```python
from build123d import *

# Parameters (mm, degrees)
SKETCH1_W           = 24.83
SKETCH1_H           = 23.79
BOSS_EXTRUDE1_DEPTH = 1.05
BOSS_EXTRUDE2_DEPTH = 4.5
SKETCH3_W           = 21.41
SKETCH3_H           = 4.84
BOSS_EXTRUDE3_DEPTH = 2.68
SKETCH4_R           = 6.265
BOSS_EXTRUDE4_DEPTH = 2.7
SKETCH5_R           = 5
BOSS_EXTRUDE5_DEPTH = 2
SKETCH6_R           = 7.16
BOSS_EXTRUDE6_DEPTH = 3
SKETCH7_R           = 6
BOSS_EXTRUDE7_DEPTH = 0.1
DOME2_FACE_RADIUS   = 6
DOME2_HEIGHT        = 1


with BuildPart() as part:
    # Sketch1 → Boss-Extrude1 (new body)
    with BuildSketch(Plane(origin=(0, 0, 0), x_dir=(1, 0, 0), z_dir=(0, 1, 0))):
        with Locations((12.415, 11.895)):
            Rectangle(SKETCH1_W, SKETCH1_H)
    extrude(amount=BOSS_EXTRUDE1_DEPTH)

    # Sketch2 → Boss-Extrude2 (add)
    with BuildSketch(Plane(origin=(0, 1.05, 0), x_dir=(1, 0, 0), z_dir=(0, 1, 0))):
        with BuildLine():
            Line((3.745, 17.925), (5.65, 17.925))
            Line((5.65, 17.925), (5.65, 22.44))
            Line((5.65, 22.44), (19.18, 22.44))
            Line((19.18, 22.44), (19.18, 17.92))
            Line((19.18, 17.92), (21.085, 17.92))
            ThreePointArc((21.085, 17.92), (23.335, 15.67), (21.085, 13.42))
            Line((21.085, 13.42), (19.18, 13.42))
            Line((19.18, 13.42), (19.18, 8.91))
            Line((19.18, 8.91), (5.65, 8.91))
            Line((5.65, 8.91), (5.65, 13.425))
            Line((5.65, 13.425), (3.745, 13.425))
            ThreePointArc((3.745, 13.425), (1.495, 15.675), (3.745, 17.925))
        make_face()
    extrude(amount=BOSS_EXTRUDE2_DEPTH)

    # Sketch3 → Boss-Extrude3 (add)
    with BuildSketch(Plane(origin=(0, 1.05, 0), x_dir=(1, 0, 0), z_dir=(0, 1, 0))):
        with Locations((12.415, 2.92)):
            Rectangle(SKETCH3_W, SKETCH3_H)
    extrude(amount=BOSS_EXTRUDE3_DEPTH)

    # Sketch4 → Boss-Extrude4 (add)
    with BuildSketch(Plane(origin=(0, 5.55, 0), x_dir=(1, 0, 0), z_dir=(0, 1, 0))):
        with Locations(Location((12.415, 15.675, 0), (0, 0, 90))):
            Circle(SKETCH4_R)
    extrude(amount=BOSS_EXTRUDE4_DEPTH)

    # Sketch5 → Boss-Extrude5 (add)
    with BuildSketch(Plane(origin=(0, 8.25, 0), x_dir=(1, 0, 0), z_dir=(0, 1, 0))):
        with Locations(Location((12.415, 15.675, 0), (0, 0, 270))):
            Circle(SKETCH5_R)
    extrude(amount=BOSS_EXTRUDE5_DEPTH)

    # Sketch6 → Boss-Extrude6 (add)
    with BuildSketch(Plane(origin=(0, 10.25, 0), x_dir=(1, 0, 0), z_dir=(0, 1, 0))):
        with Locations(Location((12.415, 15.675, 0), (0, 0, 270))):
            Circle(SKETCH6_R)
    extrude(amount=BOSS_EXTRUDE6_DEPTH)

    # Sketch7 → Boss-Extrude7 (add)
    with BuildSketch(Plane(origin=(0, 13.25, 0), x_dir=(1, 0, 0), z_dir=(0, 1, 0))):
        with Locations(Location((12.415, 15.675, 0), (0, 0, 270))):
            Circle(SKETCH7_R)
    extrude(amount=BOSS_EXTRUDE7_DEPTH)

    # Dome2: a dome of height H over a round flat face of radius A is a cap of a sphere of radius (A * A + H * H) / (2 * H)
    dome2_r = (DOME2_FACE_RADIUS * DOME2_FACE_RADIUS + DOME2_HEIGHT * DOME2_HEIGHT) / (2 * DOME2_HEIGHT)
    dome2_base = Plane((12.415, 13.35, -15.675), z_dir=(0, 1, 0))
    with Locations(dome2_base.offset(DOME2_HEIGHT - dome2_r)):
        dome2_ball = Sphere(dome2_r, mode=Mode.PRIVATE)
    add(split(dome2_ball, bisect_by=dome2_base, keep=Keep.TOP, mode=Mode.PRIVATE))


solid = part.part
```
Check sheet for the modelled part. Datum: model origin and axes. Units: mm. A direction names the side the tool comes from. Coordinates: 2 decimals unless noted, no trailing zeros. Loops run counter-clockwise (first coordinate to the right, second up) from the corner with the lowest first, then second, coordinate; pieces in that order, holes last. Notation, with made-up numbers: M -4.5,10.5 L 42.5,10.5 A14 ccw 42.5,21.5 Z; hole C 48.25,-17.5 d5. An arc over 180 degrees is marked long. Answer as a JSON object with one key per item and string values.
1. Sectioned sample at D-D on z = -20. Record the cut outline in (x, y) (3 decimals), and give its area (3 significant figures).
Outcome:
{"outline": "M 0,0 L 24.83,0 L 24.83,1.05 L 19.18,1.05 L 19.18,5.55 L 16.948,5.55 L 16.948,8.25 L 14.924,8.25 L 14.924,10.25 L 18.121,10.25 L 18.121,13.25 L 16.574,13.25 L 16.574,13.35 A17.987 ccw 8.256,13.35 L 8.256,13.25 L 6.709,13.25 L 6.709,10.25 L 9.906,10.25 L 9.906,8.25 L 7.882,8.25 L 7.882,5.55 L 5.65,5.55 L 5.65,1.05 L 0,1.05 Z", "area": "159 mm²"}
2. Sectioned sample at C-C on x = 9.5. Record the cut outline in (y, z) (3 decimals).
Outcome:
{"outline": "M 0,-23.79 L 1.05,-23.79 L 1.05,-22.44 L 5.55,-22.44 L 5.55,-21.221 L 8.25,-21.221 L 8.25,-19.737 L 10.25,-19.737 L 10.25,-22.215 L 13.25,-22.215 L 13.25,-20.919 L 13.35,-20.919 A18.269 ccw 13.35,-10.431 L 13.25,-10.431 L 13.25,-9.135 L 10.25,-9.135 L 10.25,-11.613 L 8.25,-11.613 L 8.25,-10.129 L 5.55,-10.129 L 5.55,-8.91 L 1.05,-8.91 L 1.05,-5.34 L 3.73,-5.34 L 3.73,-0.5 L 1.05,-0.5 L 1.05,0 L 0,0 Z"}
3. Sectioned sample at A-A on y = 3.25. Record the cut outline in (x, z) (3 decimals), and give its area (3 significant figures).
Outcome:
{"outline": "M 1.71,-5.34 L 23.12,-5.34 L 23.12,-0.5 L 1.71,-0.5 Z; M 3.745,-17.925 L 5.65,-17.925 L 5.65,-22.44 L 19.18,-22.44 L 19.18,-17.92 L 21.085,-17.92 A2.25 ccw 21.085,-13.42 L 19.18,-13.42 L 19.18,-8.91 L 5.65,-8.91 L 5.65,-13.425 L 3.745,-13.425 A2.25 ccw Z", "area": "320 mm²"}
4. Sectioned sample at B-B on z = -4.75. Record the cut outline in (x, y), and give its area (3 significant figures).
Outcome:
{"outline": "M 0,0 L 24.83,0 L 24.83,1.05 L 23.12,1.05 L 23.12,3.73 L 1.71,3.73 L 1.71,1.05 L 0,1.05 Z", "area": "83.5 mm²"}
5. Access from +Z, -Z, +X, -X, +Y, -Y to the whole of each face (thin tool, end or side, straight path). Record for faces 4 (the cylindrical face through (15, 12, -9)), 5 (the flat face through (1.71, 2, -3)), 6 (the flat face through (15, 8.25, -11)).
Outcome:
{"face 4": "+Y", "face 5": "+Z, -X, +Y", "face 6": "none"}
6. Scan lines: L1, parallel to Z at x = 15.5, y = 2; L2, parallel to Y at x = 18.5, z = -16; L3, parallel to X at y = 3.5, z = -9. Record each from-to range of solid material in increasing order. Write a range as from..to.
Outcome:
{"L1": "-22.44..-8.91, -5.34..-0.5", "L2": "0..8.25, 10.25..13.25", "L3": "5.65..19.18"}
7. Release check for a two-part mould opening along Z. For faces 1 (the flat face through (8, 13.25, -20)), 2 (the cylindrical face through (12.63, 9.24, -20.67)), 3 (the cylindrical face through (1.496, 3.269, -15.626)) record: pulls with the +Z half, pulls with the -Z half, needs draft (parallel to the pull), parting line crosses it, or undercut.
Outcome:
{"face 1": "needs draft", "face 2": "parting line crosses it", "face 3": "undercut"}
8. Depth check by flat-ended pin: P1, Ø4, axis at x = 14, z = -13, coming from the +Y side; P2, Ø2, axis at y = 8, z = -12.5, coming from the +X side; P3, Ø2, axis at x = 2.5, y = 10.5, coming from the -Z side; P4, Ø2, axis at y = 3, z = -21, coming from the -X side. Enter the tip coordinate at first touch or a pass-through.
Outcome:
{"P1": "y = 14.32", "P2": "x = 18.29", "P3": "through", "P4": "x = 5.65"}
